```python
from build123d import *

# Parameters (mm, degrees)
ESBO_O1_W                = 38.5
ESBO_O1_H                = 34
RESSALTO_EXTRUS_O1_DEPTH = 2.5
ESBO_O2_W                = 2.5
ESBO_O2_H                = 6
ESBO_O2_H_2              = 5.5
RESSALTO_EXTRUS_O2_DEPTH = 10
CORTE_EXTRUS_O1_REACH    = 41.373
ESBO_O3_R                = 1.5
ESBO_O4_W                = 2.95
ESBO_O4_H                = 20
RESSALTO_EXTRUS_O3_DEPTH = 13
ESBO_O5_R                = 3.45
CORTE_EXTRUS_O2_DEPTH    = 15
FILETE1_R                = 3
FILETE2_R                = 2.5
ESBO_O7_R                = 3.45
RESSALTO_EXTRUS_O5_DEPTH = 6
ESBO_O8_R                = 1.6
CORTE_EXTRUS_O3_DEPTH    = 6


with BuildPart() as part:
    # Esboço1 → Ressalto-extrusão1 (new body)
    with BuildSketch(Plane.XY):
        with Locations((-3.395014232, -10.289862205)):
            Rectangle(ESBO_O1_W, ESBO_O1_H)
    extrude(amount=RESSALTO_EXTRUS_O1_DEPTH)

    # Esboço2 → Ressalto-extrusão2 (add)
    with BuildSketch(Plane.XY.offset(2.5)):
        with Locations((1.584985768, 3.710137795)):
            Rectangle(ESBO_O2_W, ESBO_O2_H)
        with Locations((1.584985768, -24.539862205)):
            Rectangle(ESBO_O2_W, ESBO_O2_H_2)
    extrude(amount=RESSALTO_EXTRUS_O2_DEPTH)

    # Esboço3 → Corte-extrusão1 (cut, up to next)
    with BuildSketch(Plane(origin=(2.834985768, 0, 0), x_dir=(0, 0, -1), z_dir=(1, 0, 0)), mode=Mode.PRIVATE) as corte_extrus_o1_sk1:
        with Locations(Location((-9.5, 3.410137795, 0), (0, 0, 90))):
            Circle(ESBO_O3_R)
    corte_extrus_o1_tool1 = extrude(corte_extrus_o1_sk1.sketch, amount=-CORTE_EXTRUS_O1_REACH, mode=Mode.PRIVATE) & part.part
    # Esboço3 → Corte-extrusão1 (cut, up to next)
    with BuildSketch(Plane(origin=(2.834985768, 0, 0), x_dir=(0, 0, -1), z_dir=(1, 0, 0)), mode=Mode.PRIVATE) as corte_extrus_o1_sk2:
        with Locations(Location((-9.5, -24.489862205, 0), (0, 0, 90))):
            Circle(ESBO_O3_R)
    corte_extrus_o1_tool2 = extrude(corte_extrus_o1_sk2.sketch, amount=-CORTE_EXTRUS_O1_REACH, mode=Mode.PRIVATE) & part.part
    add(corte_extrus_o1_tool1.solids().sort_by_distance((2.834986, 3.410138, 9.5))[0], mode=Mode.SUBTRACT)
    add(corte_extrus_o1_tool2.solids().sort_by_distance((2.834986, -24.489862, 9.5))[0], mode=Mode.SUBTRACT)

    # Esboço4 → Ressalto-extrusão3 (add)
    with BuildSketch(Plane.XY.offset(2.5)):
        with Locations((-21.170014232, -17.289862205)):
            Rectangle(ESBO_O4_W, ESBO_O4_H)
    extrude(amount=RESSALTO_EXTRUS_O3_DEPTH)

    # Esboço5 → Corte-extrusão2 (cut)
    with BuildSketch(Plane.ZY.offset(22.645014232)):
        Polygon((2.5, -7.289862205), (15.222036194, -11.595443281), (15.5, -11.689515935), (15.5, -7.289862205), align=None)
        Polygon((15.222036194, -16.59994967), (2.5, -27.289862205), (15.5, -27.289862205), (15.5, -16.36638574), align=None)
        with Locations(Location((9.45, -15.089862205, 0), (0, 0, 270))):
            Circle(ESBO_O5_R)
    extrude(amount=-CORTE_EXTRUS_O2_DEPTH, mode=Mode.SUBTRACT)

    # Filete1
    filete1_edges = [part.edges().sort_by_distance(p)[0] for p in [
        (-21.170014232, -11.689515935, 15.5),
        (-21.170014232, -16.36638574, 15.5),
    ]]
    fillet(filete1_edges, radius=FILETE1_R)

    # Filete2
    # the kernel refuses this fillet: 2.5 mm, written as the material it adds along each edge
    with BuildSketch(Plane(origin=(-19.695014232, -7.289862205, 2.5), x_dir=(0, -0.32057353707536407, 0.947223631106715), z_dir=(-1, 0, 0))) as filete2_piece_1:
        with BuildLine():
            CenterArc((FILETE2_R * 0.717282002488, FILETE2_R), FILETE2_R, 198.697613514, 71.302386486)
            Line((-FILETE2_R * 0.229941628618, FILETE2_R * 0.679426462925), (0, 0))
            Line((0, 0), (FILETE2_R * 0.717282002488, 0))
        make_face()
    extrude(amount=2.95)

    # Esboço7 → Ressalto-extrusão5 (add)
    with BuildSketch(Plane.ZY.offset(22.645014232)):
        with Locations(Location((9.45, -15.089862205, 0), (0, 0, 270))):
            Circle(ESBO_O7_R)
    extrude(amount=-RESSALTO_EXTRUS_O5_DEPTH)

    # Esboço8 → Corte-extrusão3 (cut)
    with BuildSketch(Plane(origin=(0, 0, 0), x_dir=(-1, 0, 0), z_dir=(0, 0, -1))):
        with Locations((7.965014232, -19.289862205)):
            Circle(ESBO_O8_R)
        with Locations((-6.754985768, -14.739862205)):
            Circle(ESBO_O8_R)
    extrude(amount=-CORTE_EXTRUS_O3_DEPTH, mode=Mode.SUBTRACT)


solid = part.part
```
For this review, take the finished solid that the model builds, in its own axes (mm). A direction names the side the tool comes from. Round coordinates to 2 decimals unless told otherwise and drop trailing zeros. Write each loop counter-clockwise with the first axis right and the second up, starting at its lowest first coordinate (ties: lowest second). Pieces come first, ordered by that corner, then holes. Notation, with made-up numbers: (52.25, -8.5) - (67.25, -8.5) arc R16 cw to (67.25, -2.5) - close; hole circle Ø1 at (87.25, 68.5). An arc over 180 degrees is marked (long way). Answer as a JSON object with one key per item and string values.
1. Tool access review of faces 1 (the face through (2.835, 4, 7)), 2 (the face through (0.335, 4, 7)), 3 (the face through (2, -21.79, 7)): name each direction out of +Z, -Z, +X, -X, +Y, -Y from which nothing blocks a thin tool from reaching the whole face with its end or side.
Response values:
{"face 1": "+Z, +X, +Y, -Y", "face 2": "+Z, -X, +Y, -Y", "face 3": "+Z, +X"}
2. We need section A-A on z = 3. Give the boundary of the cut face in (x, y), then the cut area to 3 significant figures.
Response values:
{"outline": "(-22.65, -26.87) - (-19.7, -26.87) - (-19.7, -7) - (-22.65, -7) - close; (0.33, -27.29) - (2.83, -27.29) - (2.83, -21.79) - (0.33, -21.79) - close; (0.33, 0.71) - (2.83, 0.71) - (2.83, 6.71) - (0.33, 6.71) - close", "area": "87.4 mm2"}
3. To check wall thickness, follow line 1 along X through (y, z) = (-22, 4.25); line 2 along Z through (x, y) = (0, 0); line 3 along Z through (x, y) = (-17, -13.5). State the ranges of each line that lie inside material, in increasing order.
Response values:
{"line 1": "x = -22.65 to -19.7, 0.33 to 2.83", "line 2": "z = 0 to 2.5", "line 3": "z = 0 to 2.5, 6.39 to 12.51"}
4. We need section D-D on z = 5.25. Give the boundary of the cut face in (x, y).
Response values:
{"outline": "(-22.65, -24.98) - (-19.7, -24.98) - (-19.7, -8.22) - (-22.65, -8.22) - close; (0.33, -27.29) - (2.83, -27.29) - (2.83, -21.79) - (0.33, -21.79) - close; (0.33, 0.71) - (2.83, 0.71) - (2.83, 6.71) - (0.33, 6.71) - close"}
5. We need section C-C on y = -10.5. Give the boundary of the cut face in (x, z).
Response values:
{"outline": "(-22.65, 0) - (15.85, 0) - (15.85, 2.5) - (-19.7, 2.5) - (-19.7, 11.99) - (-22.65, 11.99) - close"}
6. For pin 1 Ø12 at (x, y) = (9.5, -6) entering from -Z; pin 2 Ø17 at (x, y) = (-3, -5.5) entering from +Z; pin 3 Ø5 at (y, z) = (3.41, 9.5) entering from +X (3 decimals); pin 4 Ø4 at (y, z) = (-15.5, 10.5) entering from +X (3 decimals), all flat-tipped, find the tip position at first contact; note any pin that passes through.
Response values:
{"pin 1": "stops at z = 0", "pin 2": "stops at z = 12.5", "pin 3": "stops at x = 2.835", "pin 4": "stops at x = -16.645"}
7. Draft analysis for pull direction X (two halves, no side actions). For faces 4 (the face through (-22.645, -13, 6)), 5 (the face through (2.835, -25, 7)), 6 (the face through (2, 0.71, 7)), 7 (the face through (7.102, -16.302, 1.232)), state which applies: +X half, -X half, draft (parallel to the pull), parting line (faces both ways), or undercut.
Response values:
{"face 4": "-X half", "face 5": "+X half", "face 6": "draft", "face 7": "undercut"}
8. We need section B-B on x = 9. Give the boundary of the cut face in (y, z).
Response values:
{"outline": "(-27.29, 0) - (6.71, 0) - (6.71, 2.5) - (-27.29, 2.5) - close"}
